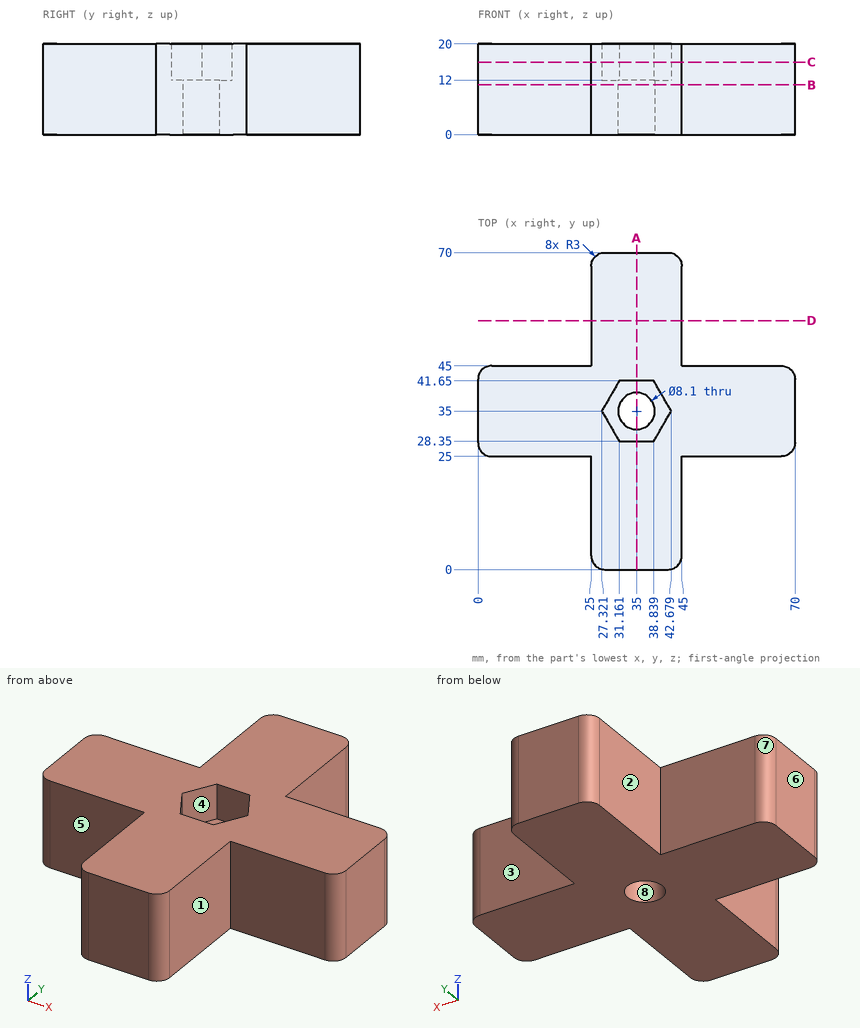
Design review of the part shown in the three views and the two pictorial views. Dimensions are in mm from the part's minimum x, y and z. A direction names the side the tool comes from. Give positions to 0.01 mm unless a question says otherwise; leave off trailing zeros. Loops run counter-clockwise (first coordinate to the right, second up) from the corner with the lowest first, then second, coordinate; pieces in that order, holes last. Notation, with made-up numbers: (86, -18.5) -> (144, -18.5) arc R15 ccw to (144, 8.5) -> close; hole circle Ø6 at (13.5, 89.25). An arc over 180 degrees is marked (long way). Answer as a JSON object with one key per item and string values. Group by question number.
Q1. Take a section at B-B (z = 11). Write out the cut boundary in (x, y), plus the area to 3 significant figures.
Q2. Wall thickness on line 1 along Y through (x, z) = (35, 6.5); line 2 along Y through (x, z) = (56, 7.25): over which ranges is each line inside the solid? List them lowest first.
Q3. Take a section at C-C (z = 16). Write out the cut boundary in (x, y).
Q4. Draft analysis for pull direction Y (two halves, no side actions). For the marked faces 6, 7 and 8, state which applies: pulls with the +Y half, pulls with the -Y half, needs draft (parallel to the pull), parting line crosses it, or undercut.
Q5. Tool access review of the marked faces 1, 2, 3, 4 and 5: name each direction out of +Z, -Z, +X, -X, +Y, -Y from which nothing blocks a thin tool from reaching the whole face with its end or side.
Q6. Take a section at A-A (x = 35). Write out the cut boundary in (y, z).
Q7. Insertion check: pin 1 (12 mm diameter, centred on y = 49, z = 16.5, fed in from +X); pin 2 (8 mm diameter, centred on x = 59, z = 9, fed in from -Y); pin 3 (6 mm diameter, centred on x = 55, z = 13.5, fed in from +Y). Each pin has a flat end and moves straight along its axis. Give the tip position at first contact, or say it passes through.
Q8. Take a section at D-D (y = 55). Write out the cut boundary in (x, z), plus the area to 3 significant figures.
Answer below:
{
 "1": {"outline": "(0, 28) arc R3 ccw to (3, 25) -> (25, 25) -> (25, 3) arc R3 ccw to (28, 0) -> (42, 0) arc R3 ccw to (45, 3) -> (45, 25) -> (67, 25) arc R3 ccw to (70, 28) -> (70, 42) arc R3 ccw to (67, 45) -> (45, 45) -> (45, 67) arc R3 ccw to (42, 70) -> (28, 70) arc R3 ccw to (25, 67) -> (25, 45) -> (3, 45) arc R3 ccw to (0, 42) -> close; hole circle Ø8.1 at (35, 35)", "area": "2,330 mm2"},
 "2": {"line 1": "y = 0 to 30.95, 39.05 to 70", "line 2": "y = 25 to 45"},
 "3": {"outline": "(0, 28) arc R3 ccw to (3, 25) -> (25, 25) -> (25, 3) arc R3 ccw to (28, 0) -> (42, 0) arc R3 ccw to (45, 3) -> (45, 25) -> (67, 25) arc R3 ccw to (70, 28) -> (70, 42) arc R3 ccw to (67, 45) -> (45, 45) -> (45, 67) arc R3 ccw to (42, 70) -> (28, 70) arc R3 ccw to (25, 67) -> (25, 45) -> (3, 45) arc R3 ccw to (0, 42) -> close; hole (27.32, 35) -> (31.16, 28.35) -> (38.84, 28.35) -> (42.68, 35) -> (38.84, 41.65) -> (31.16, 41.65) -> close"},
 "4": {"face 6": "needs draft", "face 7": "pulls with the +Y half", "face 8": "undercut"},
 "5": {"face 1": "+Z, -Z, +X, -Y", "face 2": "+Z, -Z, -X, +Y", "face 3": "+Z, -Z, +X, +Y", "face 4": "+Z", "face 5": "+Z, -Z, -X, -Y"},
 "6": {"outline": "(0, 0) -> (30.95, 0) -> (30.95, 12) -> (28.35, 12) -> (28.35, 20) -> (0, 20) -> close; (39.05, 0) -> (70, 0) -> (70, 20) -> (41.65, 20) -> (41.65, 12) -> (39.05, 12) -> close"},
 "7": {"pin 1": "stops at x = 69.83", "pin 2": "stops at y = 25", "pin 3": "stops at y = 45"},
 "8": {"outline": "(25, 0) -> (45, 0) -> (45, 20) -> (25, 20) -> close", "area": "400 mm2"}
}
